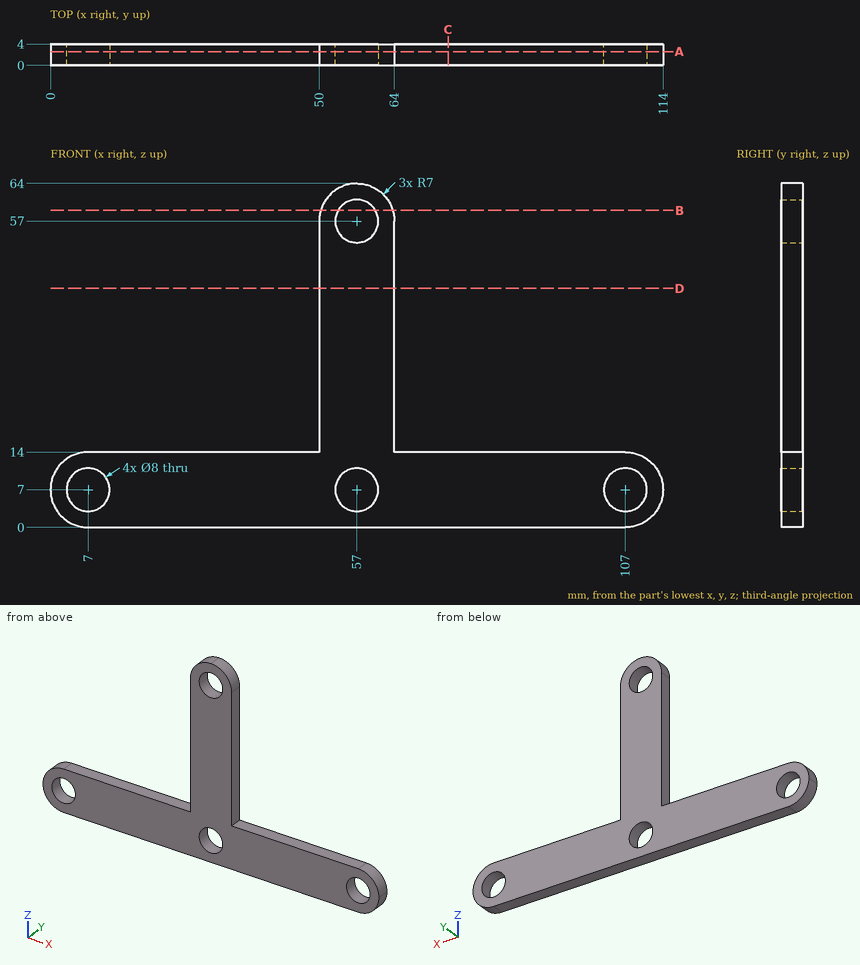
Part print with two shaded views. Sizes in mm from the minimum x, y, z corner. Round coordinates to 2 decimals unless told otherwise and drop trailing zeros. Loops run counter-clockwise (first coordinate to the right, second up) from the corner with the lowest first, then second, coordinate; pieces in that order, holes last. Notation, with made-up numbers: M 21.25,39.5 L 53.25,39.5 A13 cw 53.25,49.5 Z; hole C 17,43.25 d11. An arc over 180 degrees is marked long. Put each result on its own line as item: value. Start each with the question number.
Item 1: Cut at A-A (y = 2.6). Give the number of separate pieces and of enclosed holes in the cut face, then the cut area to 3 significant figures.
Item 2: Cut at C-C (x = 74). List the corners of the cut face in (y, z).
Item 3: Cut at B-B (z = 59). List the corners of the cut face in (x, y), then the cut area to 3 significant figures.
Item 4: Drill centre lines: line 1 along Z through (x, y) = (57, 2.2); line 2 along Z through (x, y) = (7, 2.45); line 3 along Z through (x, y) = (74.5, 1.55). Where is each one in solid material? Low to high.
Item 5: Cut at D-D (z = 44.5). List the corners of the cut face in (x, y).
Item 6: Drop flat-ended pins along their axis: P1, Ø1.2, axis at y = 2.5, z = 44, coming from the -X side; P2, Ø2, axis at x = 30.5, y = 2.5, coming from the +Z side; P3, Ø1.2, axis at y = 3, z = 40.5, coming from the +X side. Give the stop position or say it passes through.
Answer block:
1. separate pieces: 1
1. enclosed holes: 4
1. area: 2,030 mm2
2. outline: M 0,0 L 4,0 L 4,14 L 0,14 Z
3. outline: M 50.29,0 L 53.54,0 L 53.54,4 L 50.29,4 Z; M 60.46,0 L 63.71,0 L 63.71,4 L 60.46,4 Z
3. area: 26.0 mm2
4. line 1: 0 to 3, 11 to 53, 61 to 64
4. line 2: 0 to 3, 11 to 14
4. line 3: 0 to 14
5. outline: M 50,0 L 64,0 L 64,4 L 50,4 Z
6. P1: x = 50
6. P2: z = 14
6. P3: x = 64
